from build123d import *

# Parameters (mm, degrees)
F0_W     = 4
F0_H     = 40
F1_DEPTH = 25
F2_R     = 5
F3_R     = 2


with BuildPart() as f1:
    # F0 (on Top) → F1 (new body)
    with BuildSketch(Plane.XY):
        with BuildLine():
            Line((7.5, -25), (7.5, 25))
            Line((7.5, 25), (-7.5, 25))
            Line((-7.5, 25), (-7.5, -25))
            ThreePointArc((-7.5, -25), (-15.5, -33), (-23.5, -25))
            Line((-23.5, -25), (-23.5, 0))
            Line((-23.5, 0), (-34.5, 0))
            Line((-34.5, 0), (-34.5, -25))
            ThreePointArc((-34.5, -25), (-13.5, -46), (7.5, -25))
        make_face()
        Rectangle(F0_W, F0_H, mode=Mode.SUBTRACT)
    extrude(amount=F1_DEPTH)

    # F2
    f2_edges = [f1.edges().sort_by_distance(p)[0] for p in [
        (-7.5, 25, 12.5),
        (7.5, 25, 12.5),
        (-23.5, 0, 12.5),
        (-34.5, 0, 12.5),
    ]]
    fillet(f2_edges, radius=F2_R)

    # F3
    f3_edges = [f1.edges().sort_by_distance(p)[0] for p in [
        (7.5, -2.5, 25),
        (6.035534, 23.535534, 25),
        (-13.5, -46, 25),
        (0, 25, 25),
        (-34.5, -15, 25),
        (-6.035534, 23.535534, 25),
        (-33.035534, -1.464466, 25),
        (-7.5, -2.5, 25),
        (-29, 0, 25),
        (-15.5, -33, 25),
        (-24.964466, -1.464466, 25),
        (-23.5, -15, 25),
        (2, 0, 25),
        (0, -20, 25),
        (-2, 0, 25),
        (0, 20, 25),
        (7.5, -2.5, 0),
        (6.035534, 23.535534, 0),
        (-13.5, -46, 0),
        (0, 25, 0),
        (-34.5, -15, 0),
        (-6.035534, 23.535534, 0),
        (-33.035534, -1.464466, 0),
        (-7.5, -2.5, 0),
        (-29, 0, 0),
        (-15.5, -33, 0),
        (-24.964466, -1.464466, 0),
        (-23.5, -15, 0),
        (2, 0, 0),
        (0, -20, 0),
        (-2, 0, 0),
        (0, 20, 0),
    ]]
    fillet(f3_edges, radius=F3_R)


solid = f1.part
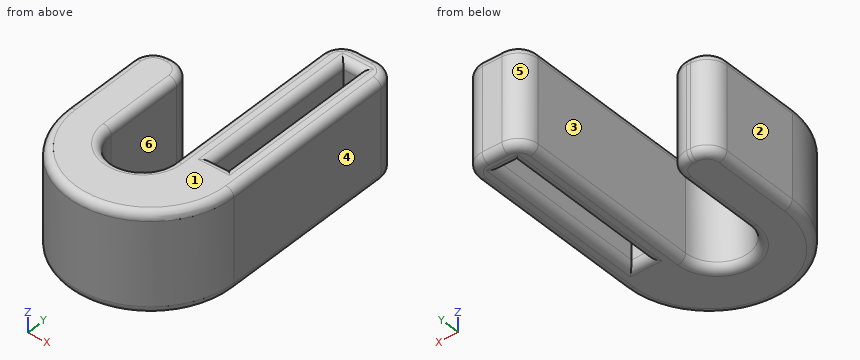
Work out the finished part from the listing and answer in its coordinate system (mm). Face numbers are marked on the shaded views. A direction names the side the tool comes from. Give positions to 0.01 mm unless a question says otherwise; leave off trailing zeros. Write each loop counter-clockwise with the first axis right and the second up, starting at its lowest first coordinate (ties: lowest second). Pieces come first, ordered by that corner, then holes.
Q1. Straight lines are drawn through the part: L1, parallel to X at y = -8.5, z = 5.25; L2, parallel to X at y = -23, z = 2.25; L3, parallel to X at y = 1.5, z = 17. For each, find the intervals that lie inside material, in ascending order.
Answer:
L1: x = -34.5 to -23.5, -7.5 to -2, 2 to 7.5
L2: x = -34.5 to -23.5, -7.5 to 7.5
L3: x = -7.5 to -2, 2 to 7.5
Q2. The part is cut by section B-B on z = 17.25. Give the vertices of the cut face in (x, y), and give its area (3 significant figures).
Answer:
outline: (-34.5, -25) arc R21 ccw to (7.5, -25) - (7.5, 20) arc R5 ccw to (2.5, 25) - (-2.5, 25) arc R5 ccw to (-7.5, 20) - (-7.5, -25) arc R8 cw to (-23.5, -25) - (-23.5, -5) arc R5 ccw to (-28.5, 0) - (-29.5, 0) arc R5 ccw to (-34.5, -5) - close; hole (-2, -20) - (2, -20) - (2, 20) - (-2, 20) - close
area: 1,440 mm2
Q3. Given pin 1 (3 mm diameter, centred on x = -21, y = -24, fed in from -Z); pin 2 (3 mm diameter, centred on x = -28, z = 11.5, fed in from -Y); pin 3 (2 mm diameter, centred on x = 0, z = 13, fed in from -Y); pin 4 (12 mm diameter, centred on y = 13, z = 18.5, fed in from -X), each flat-ended and moving along its own axis, determine where each tip first touches the part or whether it passes through.
Answer:
pin 1: passes through
pin 2: stops at y = -41.49
pin 3: stops at y = -41.87
pin 4: stops at x = -7.5
Q4. For a pull along X with two mould halves and no side action, classify the marked faces 1, 2, 3 and 4 as released by +X, released by -X, zero draft, split by the parting line, or undercut.
Answer:
face 1: zero draft
face 2: released by -X
face 3: undercut
face 4: released by +X
Q5. The part is cut by section A-A on y = 12. Give the vertices of the cut face in (x, z), and give its area (3 significant figures).
Answer:
outline: (-7.5, 2) arc R2 ccw to (-5.5, 0) - (-4, 0) arc R2 ccw to (-2, 2) - (-2, 23) arc R2 ccw to (-4, 25) - (-5.5, 25) arc R2 ccw to (-7.5, 23) - close; (2, 2) arc R2 ccw to (4, 0) - (5.5, 0) arc R2 ccw to (7.5, 2) - (7.5, 23) arc R2 ccw to (5.5, 25) - (4, 25) arc R2 ccw to (2, 23) - close
area: 268 mm2
Q6. A tool of negligible diameter and unlimited length cuts with its end or side. For the marked faces 5 and 6, from which of +Z, -Z, +X, -X, +Y, -Y can it reach the whole face along a straight path? Write none if from no direction.
Answer:
face 5: +Z, -Z, -X, +Y
face 6: +Z, -Z, +Y
